Could you check a few things on this model? Use its own coordinates, in mm. A direction names the side the tool comes from. Coordinates: 2 decimals unless noted, no trailing zeros. Loops run counter-clockwise (first coordinate to the right, second up) from the corner with the lowest first, then second, coordinate; pieces in that order, holes last. Notation, with made-up numbers: (33.5, -14.5) - (52.5, -14.5) arc R35 cw to (52.5, 17.5) - close; hole circle Ø7 at (50.5, -4). An arc over 180 degrees is marked (long way). One line per item, written item: value. Start each with the question number.
(1) I'm going to push flat-ended pins straight in: P1, Ø2, axis at x = 11, z = 12, coming from the -Y side; P2, Ø3, axis at x = 1, z = -1, coming from the +Y side; P3, Ø1.5, axis at x = 1, y = -8, coming from the +Z side; P4, Ø1.5, axis at x = 7.5, z = -9.5, coming from the -Y side. Where does each tip first touch, or does it pass through?
(2) If we section it at C-C on x = 2: Write out the boundary of the cut face in (y, z) (3 decimals).
(3) If I drill on line 1 along X through (y, z) = (0, 6.75); line 2 along Z through (x, y) = (3, -1); line 3 along Y through (x, z) = (7, -1.5), over which ranges is the centre line in solid material (lowest first)? Write a range as from..to.
(4) On a 3-axis mill with a long thin cutter (end or side, diameter ignored), from which of +Z, -Z, +X, -X, +Y, -Y can I reach the whole of each face in a straight line? I mean faces 1 (the face through (7.394, -8, -8)), 2 (the face through (6.685, 5.245, 16.656)), 3 (the face through (2.47, 13.6, 4.28)). Say none if no direction works.
(5) If we section it at A-A on y = 0: Write out the boundary of the cut face in (x, z) (1 decimal).
(6) If we mould it in two halves opening along Y, with no side actions, what happens to faces 4 (the face through (5.92, 0.95, 3.03)), 5 (the face through (2.8, 13.6, 4.3)), 6 (the face through (13.744, 0, -4))? For each: pulls with the +Y half, pulls with the -Y half, needs draft (parallel to the pull), parting line crosses it, or undercut.
(7) If we section it at B-B on z = 0: Write out the boundary of the cut face in (x, y) (1 decimal), then the cut area to 3 significant figures.
(8) If we section it at D-D on x = 4.5: Write out the boundary of the cut face in (y, z) (3 decimals).
```python
from build123d import *

# Parameters (mm, degrees)
F4_DEPTH = 27.0135


with BuildPart() as f1:
    # F0 (on Front) → F1 (revolve)
    with BuildSketch(Plane.XZ):
        Polygon((-2.131164, 3.175), (13.743836, 3.175), (13.743836, 9.525), (7.393836, 9.525), (7.393836, 17.4625), (-2.131164, 17.4625), align=None)
    revolve(axis=Axis((-0.144044, 0, 0), (-1, 0, 0)))

    # F3 (on offset) → F4 (cut, through all)
    with BuildSketch(Plane.XY.offset(9.55)):
        with BuildLine():
            Line((9.568836, 0), (11.568836, 0))
            ThreePointArc((11.568836, 0), (10.568836, 1), (9.568836, 0))
        make_face()
        with BuildLine():
            ThreePointArc((9.568836, 0), (10.568836, -1), (11.568836, 0))
            Line((11.568836, 0), (9.568836, 0))
        make_face()
    extrude(amount=-F4_DEPTH, mode=Mode.SUBTRACT)

    # F6 (on Top) → F7 (revolve, cut)
    with BuildSketch(Plane.XY):
        Polygon((5.996475, 17.4625), (-0.733803, 17.4625), (2.631336, 14.097361), align=None)
    revolve(axis=Axis((5.807324, 0, 0), (1, 0, 0)), mode=Mode.SUBTRACT)


solid = f1.part
```
Values:
1. P1: passes through
1. P2: stops at y = 17.2
1. P3: stops at z = 14.5
1. P4: stops at y = -15.11
2. outline: circle Ø29.457 at (0, 0); hole circle Ø6.35 at (0, 0)
3. line 1: x = -2.13..9.57, 11.57..13.74
3. line 2: z = -14.43..-3.01, 3.01..14.43
3. line 3: y = -17.4..-2.8, 2.8..17.4
4. face 1: +X
4. face 2: +X, -X
4. face 3: none
5. outline: (-2.1, -17.5) - (-0.7, -17.5) - (2.6, -14.1) - (6, -17.5) - (7.4, -17.5) - (7.4, -9.5) - (9.6, -9.5) - (9.6, -3.2) - (-2.1, -3.2) - close; (-2.1, 3.2) - (9.6, 3.2) - (9.6, 9.5) - (7.4, 9.5) - (7.4, 17.5) - (6, 17.5) - (2.6, 14.1) - (-0.7, 17.5) - (-2.1, 17.5) - close; (11.6, -9.5) - (13.7, -9.5) - (13.7, -3.2) - (11.6, -3.2) - close; (11.6, 3.2) - (13.7, 3.2) - (13.7, 9.5) - (11.6, 9.5) - close
6. face 4: undercut
6. face 5: parting line crosses it
6. face 6: needs draft
7. outline: (-2.1, -17.5) - (-0.7, -17.5) - (2.6, -14.1) - (6, -17.5) - (7.4, -17.5) - (7.4, -9.5) - (13.7, -9.5) - (13.7, -3.2) - (-2.1, -3.2) - close; (-2.1, 3.2) - (13.7, 3.2) - (13.7, 9.5) - (7.4, 9.5) - (7.4, 17.5) - (6, 17.5) - (2.6, 14.1) - (-0.7, 17.5) - (-2.1, 17.5) - close
7. area: 330 mm2
8. outline: circle Ø31.932 at (0, 0); hole circle Ø6.35 at (0, 0)
